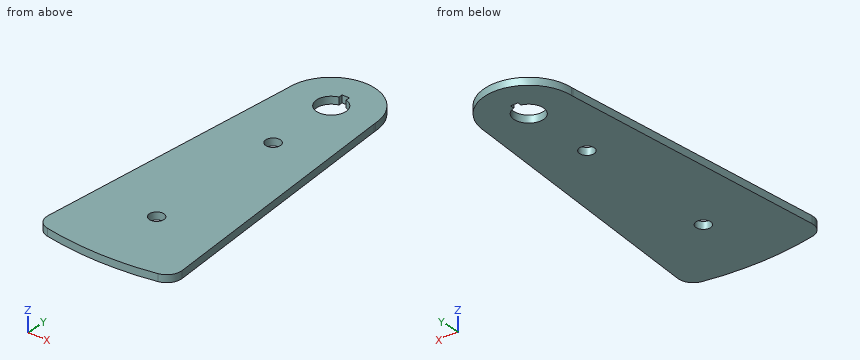
```python
from build123d import *

# Parameters (mm, degrees)
SKETCH1_R               = 12.7
BOSS_EXTRUDE1_DEPTH     = 3.175
SKETCH8_W               = 6.35
SKETCH8_H               = 6.35
CUT_EXTRUDE1_DEPTH      = 4.175
CUT_EXTRUDE1_DEPTH_BACK = 4.175
SKETCH9_R               = 6.35
CUT_EXTRUDE2_DEPTH      = 4.175
CUT_EXTRUDE2_DEPTH_BACK = 4.175
FILLET1_R               = 12.7


with BuildPart() as part:
    # Sketch1 → Boss-Extrude1 (new body, symmetric)
    with BuildSketch(Plane.XY):
        with BuildLine():
            Line((-59.699595301, -246.884504011), (-38.184359795, -0.964236874))
            ThreePointArc((-38.184359795, -0.964236874), (-38.124009824, -0.108037848), (-38.092623076, 0.749711395))
            ThreePointArc((-38.092623076, 0.749711395), (0, 38.1), (38.092623076, 0.749711395))
            ThreePointArc((38.092623076, 0.749711395), (38.124009824, -0.108037848), (38.184359795, -0.964236874))
            Line((38.184359795, -0.964236874), (59.699595301, -246.884504011))
            ThreePointArc((59.699595301, -246.884504011), (0, -254), (-59.699595301, -246.884504011))
        make_face()
        Circle(SKETCH1_R, mode=Mode.SUBTRACT)
    extrude(amount=BOSS_EXTRUDE1_DEPTH, both=True)

    # Sketch8 → Cut-Extrude1 (cut, two sides)
    with BuildSketch(Plane.XY) as cut_extrude1_sk:
        with Locations((0, 12.7)):
            Rectangle(SKETCH8_W, SKETCH8_H)
    extrude(amount=CUT_EXTRUDE1_DEPTH, mode=Mode.SUBTRACT)
    extrude(cut_extrude1_sk.sketch, amount=-CUT_EXTRUDE1_DEPTH_BACK, mode=Mode.SUBTRACT)

    # Sketch9 → Cut-Extrude2 (cut, two sides)
    with BuildSketch(Plane.XY) as cut_extrude2_sk:
        with Locations((0, -63.5)):
            Circle(SKETCH9_R)
        with Locations((0, -190.5)):
            Circle(SKETCH9_R)
    extrude(amount=CUT_EXTRUDE2_DEPTH, mode=Mode.SUBTRACT)
    extrude(cut_extrude2_sk.sketch, amount=-CUT_EXTRUDE2_DEPTH_BACK, mode=Mode.SUBTRACT)

    # Fillet1
    fillet1_edges = [part.edges().sort_by_distance(p)[0] for p in [
        (-59.699595301, -246.884504011, 0),
        (59.699595301, -246.884504011, 0),
    ]]
    fillet(fillet1_edges, radius=FILLET1_R)


solid = part.part
```
Source: CAD feature listing. Evaluate the final solid. Frame: model axes, mm. Coordinates: 2 decimals unless noted, no trailing zeros. Loops run counter-clockwise (first coordinate to the right, second up) from the corner with the lowest first, then second, coordinate; pieces in that order, holes last. Notation, with made-up numbers: M 23,38 L 27,38 A17 cw 27,71 Z; hole C -33,72 d11. An arc over 180 degrees is marked long. Use a Markdown table: item, result. Add a question column.
Q1. Section query C-C, the plane y = -63.5. Return loops of the section in (x, z) (3 decimals).
Q2. First-contact query: pin 1 (1.8 mm diameter, centred on y = 14.5, z = 0, fed in from -X); pin 2 (7.5 mm diameter, centred on x = 0, y = -190.5, fed in from +Z); pin 3 (1 mm diameter, centred on y = -176, z = 1.5, fed in from +X); pin 4 (1 mm diameter, centred on y = -121.5, z = 0.5, fed in from -X). Flat tips, straight axial feed; report the tip coordinate or a pass-through.
Q3. Section query D-D, the plane y = -190.5. Return loops of the section in (x, z) (3 decimals).
Q4. Section query B-B, the plane x = 0. Return loops of the section in (y, z) (3 decimals).
Q5. Material intervals for L1, parallel to X at y = 0, z = -2; L2, parallel to Y at x = 1, z = 0.25 (3 decimals); L3, parallel to X at y = -237, z = -0.75, sorted ascending.
Q6. Section query A-A, the plane z = 1.75. Return loops of the section in (x, y) (3 decimals).
Result:
| question | item | result |
|---|---|---|
| 1 | outline | M -43.656,-3.175 L -6.35,-3.175 L -6.35,3.175 L -43.656,3.175 Z; M 6.35,-3.175 L 43.656,-3.175 L 43.656,3.175 L 6.35,3.175 Z |
| 2 | pin 1 | stops at x = -35.59 |
| 2 | pin 2 | passes through |
| 2 | pin 3 | stops at x = 53.54 |
| 2 | pin 4 | stops at x = -48.77 |
| 3 | outline | M -54.767,-3.175 L -6.35,-3.175 L -6.35,3.175 L -54.767,3.175 Z; M 6.35,-3.175 L 54.767,-3.175 L 54.767,3.175 L 6.35,3.175 Z |
| 4 | outline | M -254,-3.175 L -196.85,-3.175 L -196.85,3.175 L -254,3.175 Z; M -184.15,-3.175 L -69.85,-3.175 L -69.85,3.175 L -184.15,3.175 Z; M -57.15,-3.175 L -12.7,-3.175 L -12.7,3.175 L -57.15,3.175 Z; M 15.875,-3.175 L 38.1,-3.175 L 38.1,3.175 L 15.875,3.175 Z |
| 5 | L1 | x = -38.12 to -12.7, 12.7 to 38.12 |
| 5 | L2 | y = -253.998 to -196.771, -184.229 to -69.771, -57.229 to -12.661, 15.875 to 38.087 |
| 5 | L3 | x = -58.77 to 58.77 |
| 6 | outline | M -58.726,-235.754 A12.7 ccw -48.499,-249.327 A254 ccw 48.499,-249.327 A12.7 ccw 58.726,-235.754 L 38.184,-0.964 A25.4 cw 38.093,0.75 A38.1 ccw -38.093,0.75 A25.4 cw -38.184,-0.964 Z; hole C 0,-190.5 d12.7; hole C 0,-63.5 d12.7; hole M -3.175,12.297 A12.7 ccw long 3.175,12.297 L 3.175,15.875 L -3.175,15.875 Z |
